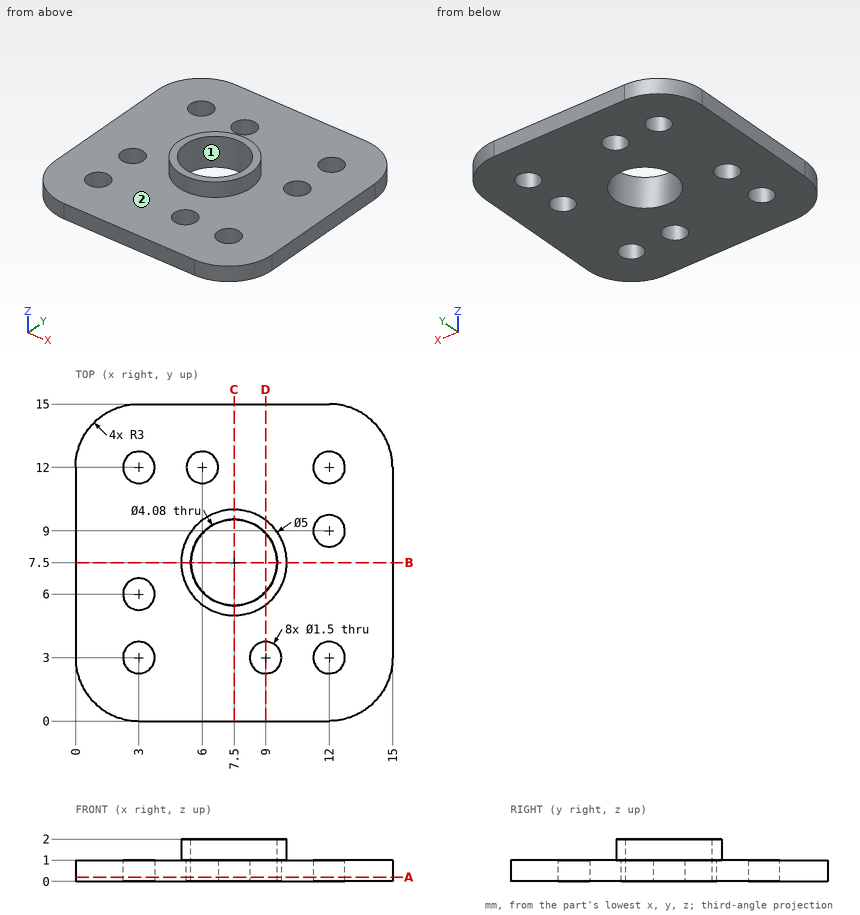
Can you work these out from the drawing? Everything is in mm from the part's minimum corner. Coordinates: 2 decimals unless noted, no trailing zeros. Order: outer loops, then holes, each group sorted by start corner. A loop starts at its lowest first (then second) coordinate and runs counter-clockwise, first axis right, second up. Notation, with made-up numbers: (21, -7.75) -> (80, -7.75) arc R27 cw to (80, 9.25) -> close; hole circle Ø6 at (-18, -25.75). An arc over 180 degrees is marked (long way). Return JSON: item names as keys, results as strings.
1) I'm going to push a flat-ended pin straight in: P1, Ø2, axis at x = 12, y = 10, coming from the +Z side. Where does the tip first touch, or does it pass through?
Conclusion:
{"P1": "stops at z = 1"}
2) If I drill on probe 1 along Y at (x, z) = (3, 0.35); probe 2 along X at (y, z) = (3, 0.7); probe 3 along Y at (x, z) = (7.5, 1.25), over which ranges is the centre line in solid material (lowest first)?
Conclusion:
{"probe 1": "y = 0 to 2.25, 3.75 to 5.25, 6.75 to 11.25, 12.75 to 15", "probe 2": "x = 0 to 2.25, 3.75 to 8.25, 9.75 to 11.25, 12.75 to 15", "probe 3": "y = 5 to 5.46, 9.54 to 10"}
3) Thinking about a two-plate mould opening in X: for the marked faces 1 and 2, which applies, +X half, -X half, draft (parallel to the pull), parting line (faces both ways), or undercut?
Conclusion:
{"face 1": "undercut", "face 2": "draft"}
4) If we section it at A-A on z = 0.2: State how many separate pieces and enclosed holes the cut face has, plus the area to 3 significant figures.
Conclusion:
{"separate pieces": "1", "enclosed holes": "9", "area": "190 mm²"}
5) If we section it at D-D on x = 9: List the corners of the cut face in (y, z) for me, plus the area to 3 significant figures.
Conclusion:
{"outline": "(0, 0) -> (2.25, 0) -> (2.25, 1) -> (0, 1) -> close; (3.75, 0) -> (6.12, 0) -> (6.12, 2) -> (5.5, 2) -> (5.5, 1) -> (3.75, 1) -> close; (8.88, 0) -> (15, 0) -> (15, 1) -> (9.5, 1) -> (9.5, 2) -> (8.88, 2) -> close", "area": "12.0 mm²"}
6) If we section it at B-B on y = 7.5: List the corners of the cut face in (x, z) for me, plus the area to 3 significant figures.
Conclusion:
{"outline": "(0, 0) -> (5.46, 0) -> (5.46, 2) -> (5, 2) -> (5, 1) -> (0, 1) -> close; (9.54, 0) -> (15, 0) -> (15, 1) -> (10, 1) -> (10, 2) -> (9.54, 2) -> close", "area": "11.8 mm²"}
